```python
from build123d import *

# Parameters (mm, degrees)
BOSS_EXTRUDE6_DEPTH = 1.27
BOSS_EXTRUDE7_DEPTH = 0.635
BOSS_EXTRUDE8_DEPTH = 2.54


with BuildPart() as part:
    # Sketch1 → Boss-Extrude6 (new body)
    with BuildSketch(Plane(origin=(0, 0, 0), x_dir=(1, 0, 0), z_dir=(0, 1, 0))):
        with BuildLine():
            Line((-9.304269575, -27.345620797), (13.511541223, -27.345620797))
            add(Edge.make_bspline(
                [(22.920452389, 30.489026504), (55.478836557, -0.15547818), (13.511541223, -27.345620797)],
                knots=[0, 0, 0, 1, 1, 1], degree=2))
            Line((22.920452389, 30.489026504), (-18.713180741, 30.489026504))
            add(Edge.make_bspline(
                [(-18.713180741, 30.489026504), (-51.271564909, -0.15547818), (-9.304269575, -27.345620797)],
                knots=[0, 0, 0, 1, 1, 1], degree=2))
        make_face()
    extrude(amount=BOSS_EXTRUDE6_DEPTH)

    # Sketch2 → Boss-Extrude7 (add)
    # profile 1 of 2: a face of its own
    with BuildSketch(Plane(origin=(0, 1.27, 0), x_dir=(1, 0, 0), z_dir=(0, 1, 0))):
        with BuildLine():
            Line((-9.304269575, -27.345620797), (13.511541223, -27.345620797))
            add(Edge.make_bspline(
                [(13.511541223, -27.345620797), (55.478836557, -0.15547818), (22.920452389, 30.489026504)],
                knots=[0, 0, 0, 1, 1, 1], degree=2))
            Line((22.920452389, 30.489026504), (-18.713180741, 30.489026504))
            add(Edge.make_bspline(
                [(-18.713180741, 30.489026504), (-51.271564909, -0.15547818), (-9.304269575, -27.345620797)],
                knots=[0, 0, 0, 1, 1, 1], degree=2))
        make_face()
        with BuildLine():
            Line((-17.979945899, 29.219026504), (22.187217547, 29.219026504))
            add(Edge.make_bspline(
                [(22.187217547, 29.219026504), (53.157284404, -0.080086004), (12.854748908, -26.075620797)],
                knots=[0, 0, 0, 1, 1, 1], degree=2))
            Line((12.854748908, -26.075620797), (-8.64747726, -26.075620797))
            add(Edge.make_bspline(
                [(-17.979945899, 29.219026504), (-48.950012756, -0.080086004), (-8.64747726, -26.075620797)],
                knots=[0, 0, 0, 1, 1, 1], degree=2))
        make_face(mode=Mode.SUBTRACT)
    # profile 2 of 2: a face of its own
    with BuildSketch(Plane(origin=(0, 1.27, 0), x_dir=(1, 0, 0), z_dir=(0, 1, 0))):
        with BuildLine():
            add(Edge.make_bspline(
                [(22.187217547, 29.219026504), (53.157284404, -0.080086004), (12.854748908, -26.075620797)],
                knots=[0, 0, 0, 1, 1, 1], degree=2))
            Line((12.854748908, -26.075620797), (-8.64747726, -26.075620797))
            add(Edge.make_bspline(
                [(-17.979945899, 29.219026504), (-48.950012756, -0.080086004), (-8.64747726, -26.075620797)],
                knots=[0, 0, 0, 1, 1, 1], degree=2))
            Line((-17.979945899, 29.219026504), (22.187217547, 29.219026504))
        make_face()
        with BuildLine():
            Line((-17.686651962, 28.711026504), (21.89392361, 28.711026504))
            add(Edge.make_bspline(
                [(21.89392361, 28.711026504), (52.228663543, -0.049929134), (12.592031982, -25.567620797)],
                knots=[0, 0, 0, 1, 1, 1], degree=2))
            Line((12.592031982, -25.567620797), (-8.384760334, -25.567620797))
            add(Edge.make_bspline(
                [(-17.686651962, 28.711026504), (-48.021391895, -0.049929134), (-8.384760334, -25.567620797)],
                knots=[0, 0, 0, 1, 1, 1], degree=2))
        make_face(mode=Mode.SUBTRACT)
    extrude(amount=BOSS_EXTRUDE7_DEPTH)

    # Sketch3 → Boss-Extrude8 (add)
    with BuildSketch(Plane(origin=(0, 1.905, 0), x_dir=(1, 0, 0), z_dir=(0, 1, 0))):
        with BuildLine():
            Line((22.187217547, 29.219026504), (-17.979945899, 29.219026504))
            add(Edge.make_bspline(
                [(-17.979945899, 29.219026504), (-48.950012756, -0.080086004), (-8.64747726, -26.075620797)],
                knots=[0, 0, 0, 1, 1, 1], degree=2))
            Line((-8.64747726, -26.075620797), (12.854748908, -26.075620797))
            add(Edge.make_bspline(
                [(22.187217547, 29.219026504), (53.157284404, -0.080086004), (12.854748908, -26.075620797)],
                knots=[0, 0, 0, 1, 1, 1], degree=2))
        make_face()
        with BuildLine():
            Line((-17.686651962, 28.711026504), (21.89392361, 28.711026504))
            add(Edge.make_bspline(
                [(12.592031982, -25.567620797), (52.228663543, -0.049929134), (21.89392361, 28.711026504)],
                knots=[0, 0, 0, 1, 1, 1], degree=2))
            Line((12.592031982, -25.567620797), (-8.384760334, -25.567620797))
            add(Edge.make_bspline(
                [(-17.686651962, 28.711026504), (-48.021391895, -0.049929134), (-8.384760334, -25.567620797)],
                knots=[0, 0, 0, 1, 1, 1], degree=2))
        make_face(mode=Mode.SUBTRACT)
    extrude(amount=BOSS_EXTRUDE8_DEPTH)


solid = part.part
```
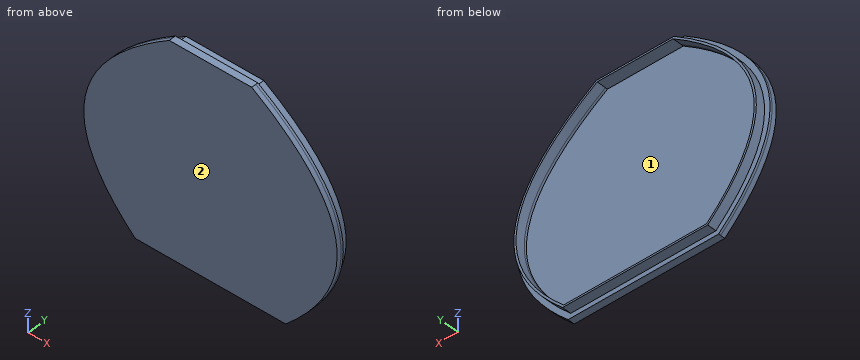
The model under review builds one solid part; all positions refer to its coordinate system, in mm. Face numbers are marked on the shaded views. Round coordinates to 2 decimals unless told otherwise and drop trailing zeros. Order: outer loops, then holes, each group sorted by start corner. A loop starts at its lowest first (then second) coordinate and runs counter-clockwise, first axis right, second up. Notation, with made-up numbers: (59, -15) - (68, -15) arc R13 ccw to (68, -10) - close; hole circle Ø3 at (6.5, 29.5). An arc over 180 degrees is marked (long way). Answer in a Markdown table with one row per item.
(1) Clearance check with flat-ended pins moving along their axes: P1, Ø1.3, axis at x = -2.5, y = 3, coming from the -Z side; P2, Ø0.8, axis at x = 5.5, y = 3, coming from the +Z side; P3, Ø1, axis at y = 2.5, z = -2, coming from the -X side. State where each tip first meets the part, or that it passes through.
Result set:
| item | result |
|---|---|
| P1 | stops at z = -29.22 |
| P2 | stops at z = 26.08 |
| P3 | stops at x = -31.36 |
(2) Mouldability with a two-part tool opening along X and no side actions: class the marked faces 1 and 2 as released by +X, released by -X, zero draft, split by the parting line, or undercut.
Result set:
| item | result |
|---|---|
| face 1 | undercut |
| face 2 | zero draft |
(3) For line 1 (Z direction, x = 3, y = 3.15); line 2 (Z direction, x = -7.5, y = 1.8); line 3 (Y direction, x = 18, z = -13.5), list the stretches that pass through material, from the lowest coordinate up. Write a range as from..to.
Result set:
| item | result |
|---|---|
| line 1 | z = -29.22..-28.71, 25.57..26.08 |
| line 2 | z = -30.49..-28.71, 25.57..27.35 |
| line 3 | y = 0..1.27 |
(4) Take a section at A-A on x = 2.5. Write out the cut boundary in (y, z) (3 decimals), plus the area to 3 significant figures.
Result set:
| item | result |
|---|---|
| outline | (0, -30.489) - (1.905, -30.489) - (1.905, -29.219) - (4.445, -29.219) - (4.445, -28.711) - (1.27, -28.711) - (1.27, 25.568) - (4.445, 25.568) - (4.445, 26.076) - (1.905, 26.076) - (1.905, 27.346) - (0, 27.346) - close |
| area | 78.3 mm2 |
